Autodesk Inventor part; units mm, degrees
sketch "Sketch2" plane through (0, 0, 0) normal (1, 0, 0) x (0, 1, 0)
  line L0 (25, 25) -> (-25, 25)
  line L1 (-25, 25) -> (-25, -25)
  line L2 (-25, -25) -> (25, -25)
  line L3 (25, -25) -> (25, 25)
  line L4 (-35, 0) -> (35, 0)
  line L5 (0, 35) -> (0, -35)
  line L6 (-25, 25) -> (25, -25)
  point P0 (0, 0)
  point P1 (25, 0)
  point P2 (0, 25)
  dimension "d0" = 50
  dimension "d1" = 50
extrude "Extrusion1" add sketch "Sketch2" along normal mid plane 10 contours L6 L4 L1 | L5 L2 L1 L4 | L6 L2 L5
sketch "Sketch4" plane through (5, 0, 0) normal (1, 0, 0) x (0, 0, -1)
  line L0 (25, 25) -> (-25, -25)
  line L1 (25, -25) -> (25, 25)
  line L2 (-25, -25) -> (25, -25)
  line L3 (22, 17.7574) -> (-17.7574, -22)
  line L4 (-17.7574, -22) -> (22, -22)
  line L5 (22, -22) -> (22, 17.7574)
  point P0 (0, 0)
  dimension "d8" = 3
extrude "Extrusion2" cut sketch "Sketch4" against normal blind 7 contours L5 L4 L3
sketch "Sketch5" plane through (-5, -25, -25) normal (0, -1, 0) x (1, 0, 0)
  line L0 (5, 60) -> (5, -10)
  circle A0 centre (5, 45) radius 2.5
  line L1 (10, 50) -> (0, 50)
  circle A1 centre (5, 5) radius 2.5
  point P0 (5, 25)
  dimension "d11" = 5
  dimension "d12" = 5
  dimension "d15" = 40
extrude "Extrusion3" add sketch "Sketch5" along normal blind 5
sketch "Sketch8" plane through (-5, -25, 25) normal (0, 0.7071, 0.7071) x (1, 0, 0)
  line L0 (10, 0) -> (0, 0)
  line L1 (0, 70.7107) -> (10, 70.7107)
  circle A0 centre (5, 50.3553) radius 2.5
  line L2 (5, 84.8528) -> (5, -14.1421)
  line L3 (-2, 35.3553) -> (12, 35.3553)
  circle A1 centre (5, 20.3553) radius 2.5
  point P0 (5, 35.3553)
  dimension "d31" = 70.7107
  dimension "d32" = 5
  dimension "d34" = 15
extrude "Extrusion4" cut sketch "Sketch8" against normal blind 7
properties part number "Roof_Wall_Small"
The model under review builds one solid part; all positions refer to its coordinate system, in mm. A direction names the side the tool comes from. Round coordinates to 2 decimals unless told otherwise and drop trailing zeros. Order: outer loops, then holes, each group sorted by start corner. A loop starts at its lowest first (then second) coordinate and runs counter-clockwise, first axis right, second up. Notation, with made-up numbers: (-10.75, 27.5) - (48.25, 27.5) arc R4 cw to (48.25, 31.5) - close; hole circle Ø5 at (71, 87.5). An arc over 180 degrees is marked (long way). Use one line per item in the form item = value.
Q1. Add section A-A on x = 1.25. Give the boundary of the cut face in (y, z).
Response values:
outline = (-30, -22.17) - (-25, -22.17) - (-25, -25) - (25, -25) - (12.14, -12.14) - (10.02, -14.26) - (17.76, -22) - (-22, -22) - (-22, 17.76) - (-14.26, 10.02) - (-12.14, 12.14) - (-25, 25) - (-25, 22.17) - (-30, 22.17) - (-30, 17.83) - (-25, 17.83) - (-25, -17.83) - (-30, -17.83) - close; (-11.2, 6.95) - (6.95, -11.2) - (9.08, -9.08) - (-9.08, 9.08) - close
Q2. Add section D-D on x = -4. Give the boundary of the cut face in (y, z).
Response values:
outline = (-25, -25) - (25, -25) - (-25, 25) - close
Q3. Tool access review of faces 1 (the cylindrical face through (1.34, -27.46, 17.89)), 2 (the flat face through (-2, -11, -11)), 3 (the flat face through (0, 0, 0)): name each direction out of +Z, -Z, +X, -X, +Y, -Y from which nothing blocks a thin tool from reaching the whole face with its end or side.
Response values:
face_1 = -Y
face_2 = +X
face_3 = +Z, +X, -X, +Y
Q4. Clearance check with flat-ended pins moving along their axes: P1, Ø4, axis at x = 3.5, z = 10.5, coming from the -Y side; P2, Ø4, axis at x = -0.5, z = -16.5, coming from the +Y side. State where each tip first meets the part, or that it passes through.
Response values:
P1 = -25
P2 = 18.5
Q5. To check wall thickness, follow line 1 (X direction, y = -11.5, z = 10.5); line 2 (Z direction, x = 3, y = -12); line 3 (Z direction, x = 1.25, y = -21.5). State the ranges of each line that lie inside material, in increasing order.
Response values:
line_1 = -5 to -2.44, 2.44 to 5
line_2 = -25 to -22, 7.76 to 12
line_3 = -25 to -22, 17.26 to 21.5
Q6. Add section B-B on z = 20. Give the boundary of the cut face in (x, y).
Response values:
outline = (-5, -25) - (-2.5, -25) - (-2.5, -30) - (2.5, -30) - (2.5, -25) - (5, -25) - (5, -20) - (-5, -20) - close
Q7. Mouldability with a two-part tool opening along Y and no side actions: class faces 4 (the cylindrical face through (-0.33, -27.46, -22.48)), 5 (the flat face through (0, -30, 20)), 6 (the flat face through (1.55, -1.84, -2.4)) as pulls with the +Y half, pulls with the -Y half, needs draft (parallel to the pull), parting line crosses it, or undercut.
Response values:
face_4 = needs draft
face_5 = pulls with the -Y half
face_6 = undercut
